The listing builds one solid part. Answer for the finished solid, in the listing's coordinates (mm). Give positions to 0.01 mm unless a question says otherwise; leave off trailing zeros. Loops run counter-clockwise (first coordinate to the right, second up) from the corner with the lowest first, then second, coordinate; pieces in that order, holes last. Notation, with made-up numbers: M 44,-36.5 L 72,-36.5 A27 ccw 72,-3.5 Z; hole C -39,-4 d1. An arc over 180 degrees is marked long. One line per item, written item: value. Start each with the question number.
Q1. A cutting plane is placed at B-B, the plane z = 1.45. Determine the outline of the cut face in (x, y), and give its area (3 significant figures).
Q2. Consider L1, parallel to Y at x = 0, z = 0.7; L2, parallel to X at y = -75.5, z = 1.75; L3, parallel to X at y = 58.5, z = 0.7. Determine where each line is inside the solid, lowest interval first.
Q3. A cutting plane is placed at D-D, the plane x = 39. Determine the outline of the cut face in (y, z).
Q4. The mould has two halves that part along X. Classify faces 1 (the cylindrical face through (-54.329, -82.028, 1.232)), 2 (the cylindrical face through (34.54, -82.03, 1.23)), 3 (the cylindrical face through (-34.586, -82.075, 1.232)), 4 (the cylindrical face through (54.282, -82.075, 1.232)): +X half, -X half, draft (parallel to the pull), parting line (faces both ways), or undercut.
Q5. A cutting plane is placed at A-A, the plane x = 0. Determine the outline of the cut face in (y, z).
Q6. A cutting plane is placed at C-C, the plane y = -56. Determine the outline of the cut face in (x, z).
Q7. A flat-ended cylindrical pin translates along its axis: pin 1 (1.2 mm diameter, centred on x = 12.5, z = 1, fed in from -Y). Find the tip coordinate at first contact, or state that the pin passes through.
from build123d import *

# Parameters (mm, degrees)
F0_R     = 9.5
F1_DEPTH = 2.5


with BuildPart() as f1:
    # F0 (on Top) → F1 (new body)
    with BuildSketch(Plane.XY):
        with BuildLine():
            ThreePointArc((-14.317976, 65.921586), (-2.261677, 46.621432), (15, 61.449946))
            ThreePointArc((15, 61.449946), (14.828514, 63.711623), (14.317976, 65.921586))
            ThreePointArc((14.317976, 65.921586), (0, 76.449946), (-14.317976, 65.921586))
        make_face()
        with Locations((0, 61.449946)):
            Circle(F0_R, mode=Mode.SUBTRACT)
        with BuildLine():
            ThreePointArc((14.317976, 65.921586), (14.828514, 63.711623), (15, 61.449946))
            ThreePointArc((15, 61.449946), (-2.261677, 46.621432), (-14.317976, 65.921586))
            Line((-14.317976, 65.921586), (-55.184302, -64.930417))
            Line((-55.184302, -64.930417), (-55.184302, -79.930417))
            ThreePointArc((-55.184302, -79.930417), (-54.305622, -82.051737), (-52.184302, -82.930417))
            Line((-52.184302, -82.930417), (-36.684302, -82.930417))
            ThreePointArc((-36.684302, -82.930417), (-34.562982, -82.051737), (-33.684302, -79.930417))
            Line((-33.684302, -79.930417), (-33.684302, -64.930417))
            Line((-33.684302, -64.930417), (33.684302, -64.930417))
            Line((33.684302, -64.930417), (33.684302, -79.930417))
            ThreePointArc((33.684302, -79.930417), (34.562982, -82.051737), (36.684302, -82.930417))
            Line((36.684302, -82.930417), (52.184302, -82.930417))
            ThreePointArc((52.184302, -82.930417), (54.305622, -82.051737), (55.184302, -79.930417))
            Line((55.184302, -79.930417), (55.184302, -64.930417))
            Line((55.184302, -64.930417), (14.317976, 65.921586))
        make_face()
    extrude(amount=F1_DEPTH)


solid = f1.part
Answer block:
1. outline: M -55.18,-79.93 A3 ccw -52.18,-82.93 L -36.68,-82.93 A3 ccw -33.68,-79.93 L -33.68,-64.93 L 33.68,-64.93 L 33.68,-79.93 A3 ccw 36.68,-82.93 L 52.18,-82.93 A3 ccw 55.18,-79.93 L 55.18,-64.93 L 14.32,65.92 A15 ccw -14.32,65.92 L -55.18,-64.93 Z; hole C 0,61.45 d19
1. area: 9,800 mm^2
2. L1: -64.93 to 51.95, 70.95 to 76.45
2. L2: -55.18 to -33.68, 33.68 to 55.18
2. L3: -16.64 to -9.03, 9.03 to 16.64
3. outline: M -82.93,0 L -13.11,0 L -13.11,2.5 L -82.93,2.5 Z
4. face 1: -X half
4. face 2: undercut
4. face 3: undercut
4. face 4: +X half
5. outline: M -64.93,0 L 51.95,0 L 51.95,2.5 L -64.93,2.5 Z; M 70.95,0 L 76.45,0 L 76.45,2.5 L 70.95,2.5 Z
6. outline: M -52.4,0 L 52.4,0 L 52.4,2.5 L -52.4,2.5 Z
7. pin 1: y = -64.93
